from build123d import *

# Parameters (mm, degrees)
SKETCH1_W                        = 228.6
SKETCH1_H                        = 228.6
BOSS_EXTRUDE1_DEPTH              = 5.08
SKETCH2_R                        = 63.5
CUT_EXTRUDE1_DEPTH               = 6.08
CUT_EXTRUDE2_DEPTH               = 6.08
CIRPATTERN1_COUNT                = 4
F_3_8_0_375_DIAMETER_HOLE1_D     = 9.525
F_3_8_0_375_DIAMETER_HOLE1_DEPTH = 5.081
CIRPATTERN2_COUNT                = 4
CHAMFER1_SIZE                    = 1.27


with BuildPart() as part:
    # Sketch1 → Boss-Extrude1 (new body)
    with BuildSketch(Plane(origin=(0, 0, 0), x_dir=(1, 0, 0), z_dir=(0, 1, 0))):
        Rectangle(SKETCH1_W, SKETCH1_H)
    extrude(amount=BOSS_EXTRUDE1_DEPTH)

    # Sketch2 → Cut-Extrude1 (cut, through all)
    with BuildSketch(Plane(origin=(0, 5.08, 0), x_dir=(1, 0, 0), z_dir=(0, 1, 0))):
        Circle(SKETCH2_R)
    extrude(amount=-CUT_EXTRUDE1_DEPTH, mode=Mode.SUBTRACT)

    # Sketch3 → Cut-Extrude2 (cut, through all)
    with BuildSketch(Plane(origin=(0, 5.08, 0), x_dir=(1, 0, 0), z_dir=(0, 1, 0))):
        with BuildLine():
            Line((114.3, 114.3), (0, 114.3))
            ThreePointArc((0, 114.3), (6.410086185, 112.56361232), (11.06735431, 107.829259072))
            ThreePointArc((11.06735431, 107.829259072), (52.809318084, 52.809318084), (107.829259072, 11.06735431))
            ThreePointArc((107.829259072, 11.06735431), (112.56361232, 6.410086185), (114.3, 0))
            Line((114.3, 0), (114.3, 114.3))
        make_face()
    cut_extrude2 = extrude(amount=-CUT_EXTRUDE2_DEPTH, mode=Mode.SUBTRACT)

    # CirPattern1: Cut-Extrude2 ×4 about axis
    cirpattern1_axis = Axis((0, 0, 0), (0, 1, 0))
    for i in range(1, CIRPATTERN1_COUNT):
        add(cut_extrude2.rotate(cirpattern1_axis, i * 360 / CIRPATTERN1_COUNT), mode=Mode.SUBTRACT)

    # 3/8 (0.375) Diameter Hole1
    with Locations(Plane(origin=(0, 5.08, 0), x_dir=(1, 0, 0), z_dir=(0, 1, 0))):
        with Locations((101.6, 0)):
            f_3_8_0_375_diameter_hole1 = Hole(F_3_8_0_375_DIAMETER_HOLE1_D / 2, depth=F_3_8_0_375_DIAMETER_HOLE1_DEPTH)

    # CirPattern2: 3/8 (0.375) Diameter Hole1 ×4 about axis
    cirpattern2_axis = Axis((0, 0, 0), (0, 1, 0))
    for i in range(1, CIRPATTERN2_COUNT):
        add(f_3_8_0_375_diameter_hole1.rotate(cirpattern2_axis, i * 360 / CIRPATTERN2_COUNT), mode=Mode.SUBTRACT)

    # Chamfer1
    chamfer1_edges = [part.edges().sort_by_distance(p)[0] for p in [
        (-63.5, 0, 0),
        (-63.5, 5.08, 0),
    ]]
    chamfer(chamfer1_edges, length=CHAMFER1_SIZE)


solid = part.part
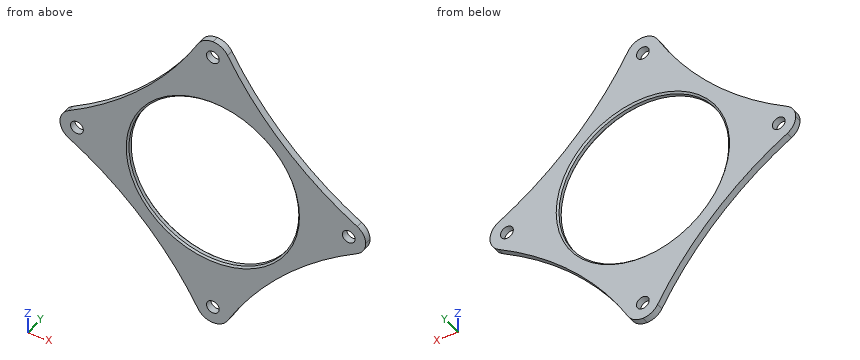
Source: CAD feature listing. Evaluate the final solid. Frame: model axes, mm. Round coordinates to 2 decimals unless told otherwise and drop trailing zeros. Loops run counter-clockwise (first coordinate to the right, second up) from the corner with the lowest first, then second, coordinate; pieces in that order, holes last. Notation, with made-up numbers: (60.25, 10.5) - (116.25, 10.5) arc R35 cw to (116.25, 47.5) - close; hole circle Ø2 at (44.25, 45). An arc over 180 degrees is marked (long way). Write item = value, one per line. Start each with the question number.
(1) Section query C-C, the plane x = 101.6. Output: boundary loops of the cut face in (y, z), plus the area to 3 significant figures.
(2) Pin query (flat end, axial travel): pin 1 (8.5 mm diameter, centred on x = -101.6, z = 0, fed in from +Y); pin 2 (1.5 mm diameter, centred on y = 2.5, z = -76, fed in from +X); pin 3 (1 mm diameter, centred on y = 2.5, z = 50, fed in from +X). Return the tip coordinate at first contact, or that it passes through.
(3) Ray query, line 1 along X through (y, z) = (2.05, 14); line 2 along Z through (x, y) = (16.5, 3); line 3 along X through (y, z) = (1.6, 101.6). Return the intervals inside material, ascending. Write a range as from..to.
(4) Section query D-D, the plane z = 78.5. Output: boundary loops of the cut face in (x, y), plus the area to 3 significant figures.
(5) Section query A-A, the plane y = 2.5. Output: boundary loops of the cut face in (x, z) (1 decimal), plus the area to 3 significant figures.
(6) Section query B-B, the plane z = 101.6. Output: boundary loops of the cut face in (x, y), plus the area to 3 significant figures.
Conclusion:
q1.outline = (0, -14.69) - (5.08, -14.69) - (5.08, -4.76) - (0, -4.76) - close; (0, 4.76) - (5.08, 4.76) - (5.08, 14.69) - (0, 14.69) - close
q1.area = 101 mm2
q2.pin_1 = through
q2.pin_2 = 32.88
q2.pin_3 = 56.18
q3.line_1 = -102.76..-61.94, 61.94..102.76
q3.line_2 = -98.63..-61.32, 61.32..98.63
q3.line_3 = -14.69..-4.76, 4.76..14.69
q4.outline = (-30.36, 0) - (30.36, 0) - (30.36, 5.08) - (-30.36, 5.08) - close
q4.area = 308 mm2
q5.outline = (-107.8, -11.1) arc R254 cw to (-11.1, -107.8) arc R12.7 ccw to (11.1, -107.8) arc R254 cw to (107.8, -11.1) arc R12.7 ccw to (107.8, 11.1) arc R254 cw to (11.1, 107.8) arc R12.7 ccw to (-11.1, 107.8) arc R254 cw to (-107.8, 11.1) arc R12.7 ccw to start; hole circle Ø9.5 at (-101.6, 0); hole circle Ø127 at (0, 0); hole circle Ø9.5 at (0, -101.6); hole circle Ø9.5 at (0, 101.6); hole circle Ø9.5 at (101.6, 0)
q5.area = 11,800 mm2
q6.outline = (-14.69, 0) - (-4.76, 0) - (-4.76, 5.08) - (-14.69, 5.08) - close; (4.76, 0) - (14.69, 0) - (14.69, 5.08) - (4.76, 5.08) - close
q6.area = 101 mm2
